```python
from build123d import *

# Parameters (mm, degrees)
F0_W     = 600
F0_H     = 400
F1_DEPTH = 1800
F2_W     = 580
F2_H     = 1780
F3_DEPTH = 390


with BuildPart() as f1:
    # F0 (on Top) → F1 (new body)
    with BuildSketch(Plane.XY):
        with Locations((190.787974, 63.787562)):
            Rectangle(F0_W, F0_H)
    extrude(amount=F1_DEPTH)

    # F2 (on face) → F3 (cut)
    with BuildSketch(Plane.XZ.offset(136.212438)):
        with Locations((190.787974, 900)):
            Rectangle(F2_W, F2_H)
    extrude(amount=-F3_DEPTH, mode=Mode.SUBTRACT)

    # F4: F1 across face


with BuildPart() as f1_1:
    add(f1.part)
    add(f1.part.mirror(Plane(origin=(190.787974, 263.787562, 900), x_dir=(-1, 0, 0), z_dir=(0, 1, 0))))


solid = f1_1.part
```
Here's how the part is built. I have some questions about the finished solid (model axes, mm). A direction names the side the tool comes from. Coordinates: 2 decimals unless noted, no trailing zeros. Order: outer loops, then holes, each group sorted by start corner. A loop starts at its lowest first (then second) coordinate and runs counter-clockwise, first axis right, second up.
Item 1: I need wall thicknesses on probe 1 along Z at (x, y) = (4.5, 340.5); probe 2 along X at (y, z) = (455, 954); probe 3 along Y at (x, z) = (121, 1467.5). Which ranges of each line are inside material? Lowest first, please.
Response values:
probe 1: z = 0 to 10, 1790 to 1800
probe 2: x = -109.21 to -99.21, 480.79 to 490.79
probe 3: y = 253.79 to 273.79
Item 2: If we section it at C-C, the plane y = -51: List the corners of the cut face in (x, z) for me, then the cut area to 3 significant figures.
Response values:
outline: (-109.21, 0) - (490.79, 0) - (490.79, 1800) - (-109.21, 1800) - close; hole (-99.21, 10) - (480.79, 10) - (480.79, 1790) - (-99.21, 1790) - close
area: 47,600 mm2
Item 3: If we section it at B-B, the plane x = 326.5: List the corners of the cut face in (y, z) for me, then the cut area to 3 significant figures.
Response values:
outline: (-136.21, 0) - (663.79, 0) - (663.79, 10) - (273.79, 10) - (273.79, 1790) - (663.79, 1790) - (663.79, 1800) - (-136.21, 1800) - (-136.21, 1790) - (253.79, 1790) - (253.79, 10) - (-136.21, 10) - close
area: 51,600 mm2
Item 4: Which directions (+Z, -Z, +X, -X, +Y, -Y) give clear straight access to the entire face, cutting with the end or side of a thin tool? Please do faces 1 (the face through (187, 56, 10)), 2 (the face through (187, 258, 0)), 3 (the face through (-99.212, 472, 888)).
Response values:
face 1: -Y
face 2: -Z, +X, -X, +Y, -Y
face 3: +Y
Item 5: If we section it at A-A, the plane z = 582: List the corners of the cut face in (x, y) for me.
Response values:
outline: (-109.21, -136.21) - (-99.21, -136.21) - (-99.21, 253.79) - (480.79, 253.79) - (480.79, -136.21) - (490.79, -136.21) - (490.79, 663.79) - (480.79, 663.79) - (480.79, 273.79) - (-99.21, 273.79) - (-99.21, 663.79) - (-109.21, 663.79) - close
Item 6: I'm going to push flat-ended pins straight in: pin 1 Ø1.5 at (x, z) = (-16, 383) entering from +Y; pin 2 Ø8 at (x, z) = (362.5, 787) entering from -Y. Where does each tip first touch, or does it pass through?
Response values:
pin 1: stops at y = 273.79
pin 2: stops at y = 253.79
Item 7: Thinking about a two-plate mould opening in Y: for faces 4 (the face through (-99.212, 56, 888)), 5 (the face through (187, 273.788, 912)), 6 (the face through (187, 253.788, 912)), which applies, pulls with the +Y half, pulls with the -Y half, needs draft (parallel to the pull), parting line crosses it, or undercut?
Response values:
face 4: needs draft
face 5: pulls with the +Y half
face 6: pulls with the -Y half
